The figure shows three views and two pictorial views of one solid part (mm, origin at its lowest corner). Answer the questions. A direction names the side the tool comes from. Round coordinates to 2 decimals unless told otherwise and drop trailing zeros. Order: outer loops, then holes, each group sorted by start corner. A loop starts at its lowest first (then second) coordinate and runs counter-clockwise, first axis right, second up. Notation, with made-up numbers: (15.5, 57) - (52.5, 57) arc R32 cw to (52.5, 91) - close; hole circle Ø7 at (2, 27.5). An arc over 180 degrees is marked (long way). One line per question, with ' | ' between items. Start each with the question number.
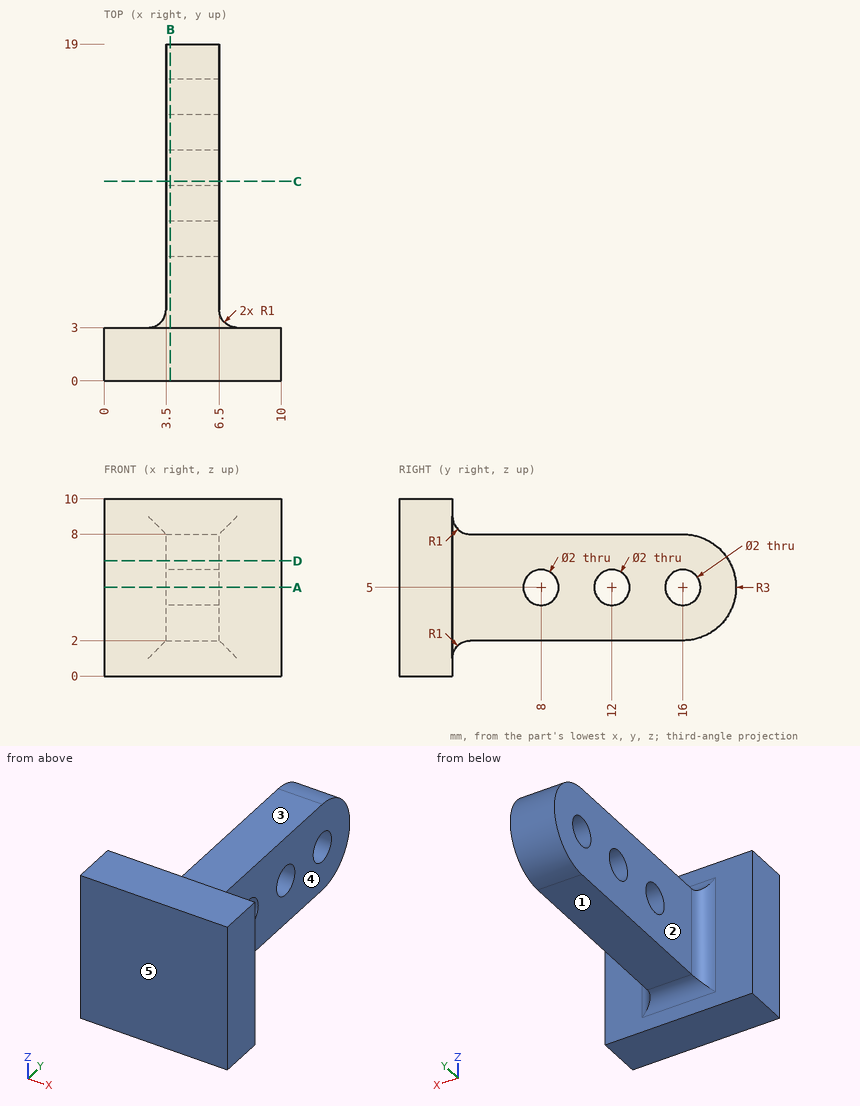
1) Flat-ended cylindrical pins translate along their axes: pin 1 (2 mm diameter, centred on y = 7, z = 4.5, fed in from -X); pin 2 (6 mm diameter, centred on x = 7.5, y = 15, fed in from +Z); pin 3 (3 mm diameter, centred on y = 12, z = 5, fed in from +X); pin 4 (5 mm diameter, centred on x = 4.5, z = 5, fed in from -Y). Find the tip coordinate at first contact, or state that the pin passes through.
2) Section A-A on z = 5 is taken. Give the vertices of the cut face in (x, y).
3) For the marked faces 1, 2, 3, 4 and 5, determine the directions among +Z, -Z, +X, -X, +Y, -Y from which every point of the face is accessible in a straight line to the end or side of a thin tool.
4) Straight lines are drawn through the part: line 1 (Y direction, x = 5.75, z = 5); line 2 (Z direction, x = 4.5, y = 10.75); line 3 (X direction, y = 17.5, z = 7.25). For each, find the intervals that lie inside material, in ascending order.
5) Section D-D on z = 6.5 is taken. Give the vertices of the cut face in (x, y), and give its area (3 significant figures).
6) Section C-C on y = 11.25 is taken. Give the vertices of the cut face in (x, z), and give its area (3 significant figures).
7) Section B-B on x = 3.75 is taken. Give the vertices of the cut face in (y, z), and give its area (3 significant figures).
Recorded:
1) pin 1: stops at x = 3.5 | pin 2: stops at z = 8 | pin 3: stops at x = 6.5 | pin 4: stops at y = 0
2) outline: (0, 0) - (10, 0) - (10, 3) - (7.5, 3) arc R1 cw to (6.5, 4) - (6.5, 7) - (3.5, 7) - (3.5, 4) arc R1 cw to (2.5, 3) - (0, 3) - close; (3.5, 9) - (6.5, 9) - (6.5, 11) - (3.5, 11) - close; (3.5, 13) - (6.5, 13) - (6.5, 15) - (3.5, 15) - close; (3.5, 17) - (6.5, 17) - (6.5, 19) - (3.5, 19) - close
3) face 1: -Z, +X, -X, +Y | face 2: +Z, -Z, -X, +Y | face 3: +Z, +X, -X, +Y | face 4: +Z, -Z, +X, +Y | face 5: +Z, -Z, +X, -X, -Y
4) line 1: y = 0 to 7, 9 to 11, 13 to 15, 17 to 19 | line 2: z = 2 to 8 | line 3: x = 3.5 to 6.5
5) outline: (0, 0) - (10, 0) - (10, 3) - (7.5, 3) arc R1 cw to (6.5, 4) - (6.5, 18.6) - (3.5, 18.6) - (3.5, 4) arc R1 cw to (2.5, 3) - (0, 3) - close | area: 77.2 mm²
6) outline: (3.5, 2) - (6.5, 2) - (6.5, 4.34) - (3.5, 4.34) - close; (3.5, 5.66) - (6.5, 5.66) - (6.5, 8) - (3.5, 8) - close | area: 14.0 mm²
7) outline: (0, 0) - (3, 0) - (3, 1) arc R1 cw to (4, 2) - (16, 2) arc R3 ccw to (16, 8) - (4, 8) arc R1 cw to (3, 9) - (3, 10) - (0, 10) - close; hole circle Ø2 at (8, 5); hole circle Ø2 at (12, 5); hole circle Ø2 at (16, 5) | area: 113 mm²
